Study the drawing (mm; zero at the part's minimum x, y, z) and answer. A direction names the side the tool comes from. Coordinates: 2 decimals unless noted, no trailing zeros. Loops run counter-clockwise (first coordinate to the right, second up) from the corner with the lowest first, then second, coordinate; pieces in that order, holes last. Notation, with made-up numbers: M 34,82.25 L 52,82.25 A15 ccw 52,90.25 Z; hole C -8.5,-16.5 d11. An arc over 180 degrees is marked long. Use one line per item in the form item = value. Start each with the question number.
1. The part is cut by section A-A (x = 88). Give the vertices of the cut face in (y, z).
2. The part is cut by section B-B (z = 7.25). Give the vertices of the cut face in (x, y), plus the area to 3 significant figures.
3. The part is cut by section D-D (x = 164.5). Give the vertices of the cut face in (y, z).
4. Find the intervals of material crossed by probe 1 along X at (y, z) = (52, 8.5); probe 2 along Z at (x, y) = (45, 73.5); probe 3 along Y at (x, z) = (98, 16.25), in increasing order. Write a range as [from, to].
5. The part is cut by section C-C (y = 63.5). Give the vertices of the cut face in (x, z) (1 decimal).
6. A tool of negligible diameter and unlimited length cuts with its end or side. For the marked faces 1 and 2, from which of +Z, -Z, +X, -X, +Y, -Y can it reach the whole face along a straight path? Write none if from no direction.
7. Flat-ended cylindrical pins translate along their axes: pin 1 (1.5 mm diameter, centred on x = 63, y = 48.5, fed in from +Z); pin 2 (10 mm diameter, centred on y = 75, z = 11, fed in from +X); pin 3 (4.5 mm diameter, centred on y = 80, z = 12.5, fed in from -X). Find the tip coordinate at first contact, or state that the pin passes through.
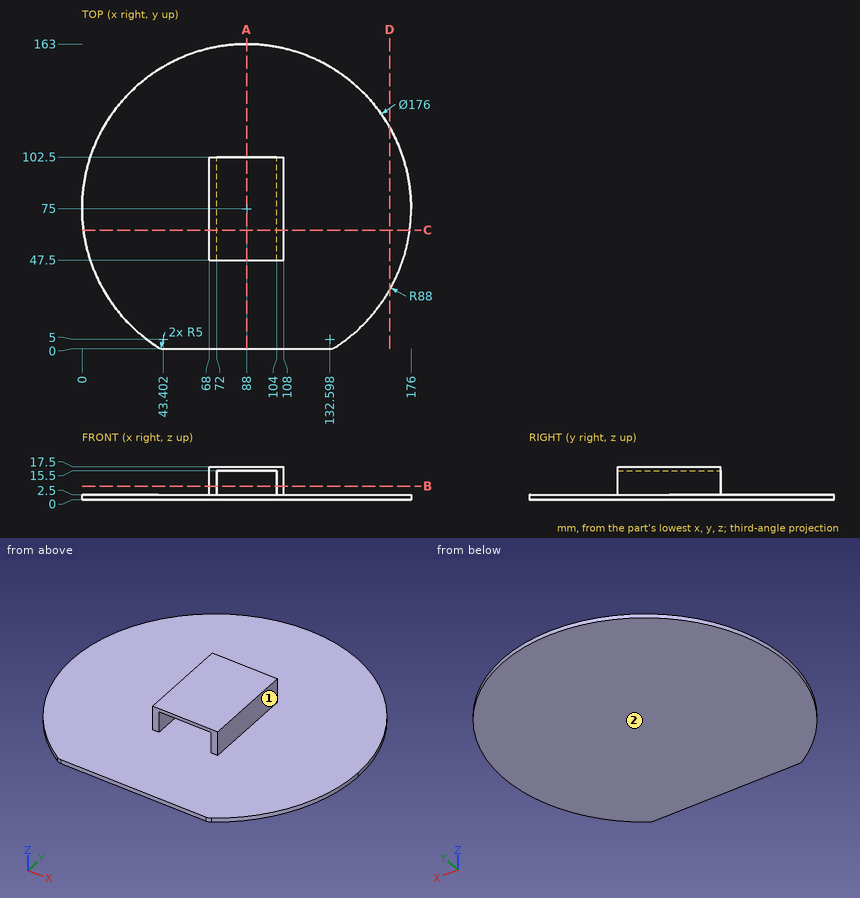
Computed values:
q1.outline = M 0,0 L 163,0 L 163,2.5 L 0,2.5 Z; M 47.5,15.5 L 102.5,15.5 L 102.5,17.5 L 47.5,17.5 Z
q2.outline = M 68,47.5 L 72,47.5 L 72,102.5 L 68,102.5 Z; M 104,47.5 L 108,47.5 L 108,102.5 L 104,102.5 Z
q2.area = 440 mm²
q3.outline = M 31.51,0 L 118.49,0 L 118.49,2.5 L 31.51,2.5 Z
q4.probe_1 = [68, 72], [104, 108]
q4.probe_2 = [0, 2.5]
q4.probe_3 = [47.5, 102.5]
q5.outline = M 0.8,0 L 175.2,0 L 175.2,2.5 L 108,2.5 L 108,17.5 L 68,17.5 L 68,2.5 L 0.8,2.5 Z; hole M 72,2.5 L 104,2.5 L 104,15.5 L 72,15.5 Z
q6.face_1 = +Z, +X, +Y, -Y
q6.face_2 = -Z, +X, -X, +Y, -Y
q7.pin_1 = 2.5
q7.pin_2 = 108
q7.pin_3 = 68
